Part print with two shaded views. Sizes in mm from the minimum x, y, z corner. A direction names the side the tool comes from. Give positions to 0.01 mm unless a question says otherwise; leave off trailing zeros. Write each loop counter-clockwise with the first axis right and the second up, starting at its lowest first coordinate (ties: lowest second). Pieces come first, ordered by that corner, then holes. Notation, with made-up numbers: (55, -5.75) -> (60, -5.75) arc R23 ccw to (60, 30.25) -> close; hole circle Ø2 at (16, 70). An arc over 180 degrees is marked (long way). Answer as a JSON object with one key per item and string values.
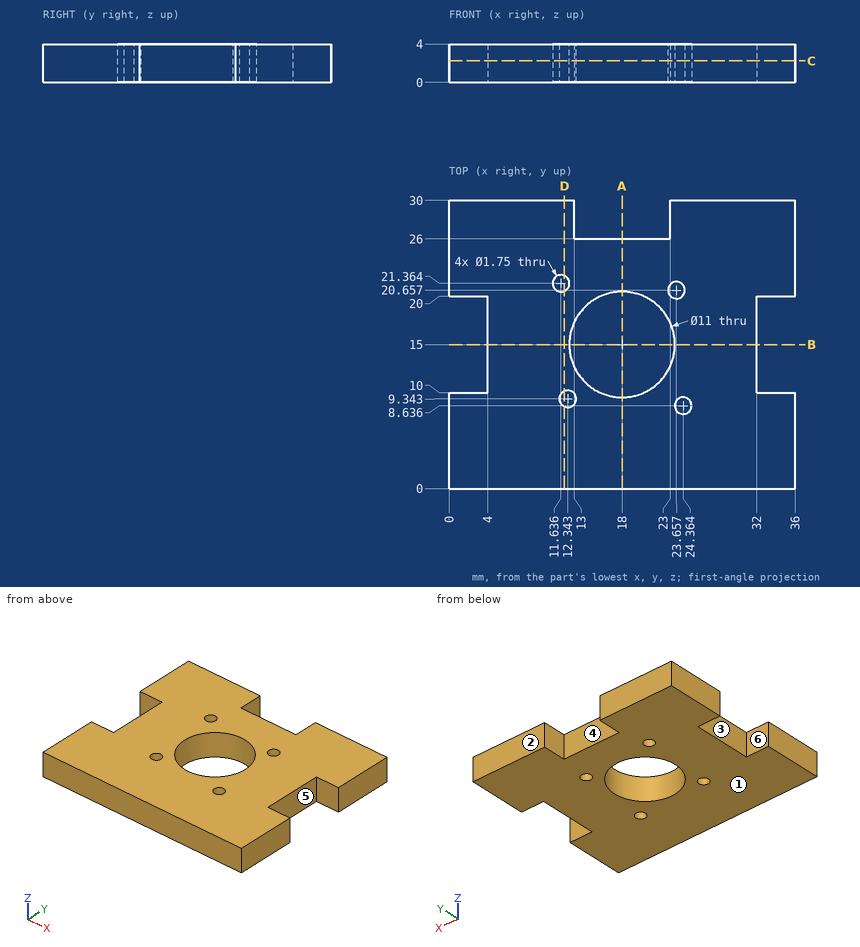
1) 3-axis set-ups, long thin cutter, end or side, ignore diameter. For the marked faces 4, 5 and 6: which of +Z, -Z, +X, -X, +Y, -Y reach the whole face in a straight line?
Model answer:
{"face 4": "+Z, -Z, +Y", "face 5": "+Z, -Z, +X", "face 6": "+Z, -Z, -X"}
2) Pin check, flat tip, straight feed: pin 1 (1.4 mm diameter, centred on x = 11.64, y = 21.36, fed in from +Z). Stop position of the tip, or through.
Model answer:
{"pin 1": "passes through"}
3) Slice it at C-C (z = 2.25). List the corners of the cut face in (x, y) (3 decimals).
Model answer:
{"outline": "(0, 0) -> (36, 0) -> (36, 10) -> (32, 10) -> (32, 20) -> (36, 20) -> (36, 30) -> (23, 30) -> (23, 26) -> (13, 26) -> (13, 30) -> (0, 30) -> (0, 20) -> (4, 20) -> (4, 10) -> (0, 10) -> close; hole circle Ø1.75 at (11.636, 21.364); hole circle Ø1.75 at (12.343, 9.343); hole circle Ø11 at (18, 15); hole circle Ø1.75 at (23.657, 20.657); hole circle Ø1.75 at (24.364, 8.636)"}
4) Mould opens along Y. For the marked faces 1, 2 and 3 say: released by +Y, released by -Y, zero draft, split by the parting line, or undercut.
Model answer:
{"face 1": "zero draft", "face 2": "released by +Y", "face 3": "undercut"}
5) Wall check: probe 1 along Y at (x, z) = (34, 1.3); probe 2 along X at (y, z) = (20.75, 3.65); probe 3 along X at (y, z) = (28, 0.65). Give the ranges that are in metal, low to high.
Model answer:
{"probe 1": "y = 0 to 10, 20 to 30", "probe 2": "x = 0 to 11.01, 12.26 to 22.79, 24.53 to 36", "probe 3": "x = 0 to 13, 23 to 36"}
6) Slice it at A-A (x = 18). List the corners of the cut face in (y, z).
Model answer:
{"outline": "(0, 0) -> (9.5, 0) -> (9.5, 4) -> (0, 4) -> close; (20.5, 0) -> (26, 0) -> (26, 4) -> (20.5, 4) -> close"}
7) Slice it at B-B (y = 15). List the corners of the cut face in (x, z), then the cut area to 3 significant figures.
Model answer:
{"outline": "(4, 0) -> (12.5, 0) -> (12.5, 4) -> (4, 4) -> close; (23.5, 0) -> (32, 0) -> (32, 4) -> (23.5, 4) -> close", "area": "68.0 mm2"}
8) Slice it at D-D (x = 12). List the corners of the cut face in (y, z).
Model answer:
{"outline": "(0, 0) -> (8.54, 0) -> (8.54, 4) -> (0, 4) -> close; (10.15, 0) -> (20.57, 0) -> (20.57, 4) -> (10.15, 4) -> close; (22.16, 0) -> (30, 0) -> (30, 4) -> (22.16, 4) -> close"}
